```python
from build123d import *

# Parameters (mm, degrees)
SKETCH1_R            = 75
BOSS_EXTRUDE1_DEPTH  = 8
M5_CLEARANCE_HOLE1_D = 5.5
CUT_EXTRUDE2_DEPTH   = 4.2
SKETCH11_R           = 45.85
CUT_EXTRUDE3_DEPTH   = 6
SKETCH12_R           = 60.7695
SKETCH12_R_2         = 53.6575
CUT_EXTRUDE4_DEPTH   = 4.1656
SKETCH14_R           = 0.5
CENTER_HOLE_DEPTH    = 1


with BuildPart() as part:
    # Sketch1 → Boss-Extrude1 (new body)
    with BuildSketch(Plane.XY):
        Circle(SKETCH1_R)
    extrude(amount=BOSS_EXTRUDE1_DEPTH)

    # M5 Clearance Hole1 (through all)
    with Locations(Plane(origin=(0, 0, 0), x_dir=(-1, 0, 0), z_dir=(0, 0, -1))):
        with Locations((-17.470285544, -65.199993275), (-47.72970773, 47.72970773), (65.199993275, -17.470285544), (47.72970773, -47.72970773), (-65.199993275, 17.470285544), (-17.470285544, 65.199993275), (-65.199993275, -17.470285544), (-47.72970773, -47.72970773), (17.470285544, -65.199993275), (65.199993275, 17.470285544), (47.72970773, 47.72970773), (17.470285544, 65.199993275)):
            Hole(M5_CLEARANCE_HOLE1_D / 2)

    # Sketch6 → Cut-Extrude2 (cut)
    with BuildSketch(Plane(origin=(0, 0, 8), x_dir=(-1, 0, 0), z_dir=(0, 0, -1))):
        Polygon((-43.268287443, 46.534273767), (-44.463721406, 50.995694054), (-48.925141693, 52.191128017), (-52.191128017, 48.925141693), (-50.995694054, 44.463721406), (-46.534273767, 43.268287443), align=None)
        Polygon((-13.008865258, 66.395427237), (-16.274851582, 69.661413561), (-20.736271868, 68.465979598), (-21.931705831, 64.004559312), (-18.665719507, 60.738572988), (-14.204299221, 61.934006951), align=None)
        Polygon((21.931705831, 64.004559312), (20.736271868, 68.465979598), (16.274851582, 69.661413561), (13.008865258, 66.395427237), (14.204299221, 61.934006951), (18.665719507, 60.738572988), align=None)
        Polygon((50.995694054, 44.463721406), (52.191128017, 48.925141693), (48.925141693, 52.191128017), (44.463721406, 50.995694054), (43.268287443, 46.534273767), (46.534273767, 43.268287444), align=None)
        Polygon((66.395427237, 13.008865258), (69.661413561, 16.274851582), (68.465979598, 20.736271868), (64.004559312, 21.931705831), (60.738572988, 18.665719507), (61.934006951, 14.204299221), align=None)
        Polygon((64.004559312, -21.931705831), (68.465979598, -20.736271868), (69.661413561, -16.274851582), (66.395427237, -13.008865258), (61.934006951, -14.204299221), (60.738572988, -18.665719507), align=None)
        Polygon((44.463721406, -50.995694054), (48.925141693, -52.191128017), (52.191128017, -48.925141693), (50.995694054, -44.463721406), (46.534273767, -43.268287443), (43.268287444, -46.534273767), align=None)
        Polygon((13.008865258, -66.395427237), (16.274851582, -69.661413561), (20.736271868, -68.465979598), (21.931705831, -64.004559312), (18.665719507, -60.738572988), (14.204299221, -61.934006951), align=None)
        Polygon((-21.931705831, -64.004559312), (-20.736271868, -68.465979598), (-16.274851582, -69.661413561), (-13.008865258, -66.395427237), (-14.204299221, -61.934006951), (-18.665719507, -60.738572988), align=None)
        Polygon((-50.995694054, -44.463721406), (-52.191128017, -48.925141693), (-48.925141693, -52.191128017), (-44.463721406, -50.995694054), (-43.268287443, -46.534273767), (-46.534273767, -43.268287443), align=None)
        Polygon((-66.395427237, -13.008865258), (-69.661413561, -16.274851582), (-68.465979598, -20.736271868), (-64.004559312, -21.931705831), (-60.738572988, -18.665719507), (-61.934006951, -14.204299221), align=None)
        Polygon((-64.004559312, 21.931705831), (-68.465979598, 20.736271868), (-69.661413561, 16.274851582), (-66.395427237, 13.008865258), (-61.934006951, 14.204299221), (-60.738572988, 18.665719507), align=None)
    extrude(amount=CUT_EXTRUDE2_DEPTH, mode=Mode.SUBTRACT)

    # Sketch11 → Cut-Extrude3 (cut)
    with BuildSketch(Plane(origin=(0, 0, 0), x_dir=(-1, 0, 0), z_dir=(0, 0, -1))):
        Circle(SKETCH11_R)
    extrude(amount=-CUT_EXTRUDE3_DEPTH, mode=Mode.SUBTRACT)

    # Sketch12 → Cut-Extrude4 (cut)
    with BuildSketch(Plane(origin=(0, 0, 0), x_dir=(-1, 0, 0), z_dir=(0, 0, -1))):
        Circle(SKETCH12_R)
        Circle(SKETCH12_R_2, mode=Mode.SUBTRACT)
    extrude(amount=-CUT_EXTRUDE4_DEPTH, mode=Mode.SUBTRACT)

    # Sketch14 → center hole (cut)
    with BuildSketch(Plane.XY.offset(8)):
        Circle(SKETCH14_R)
    extrude(amount=-CENTER_HOLE_DEPTH, mode=Mode.SUBTRACT)


solid = part.part
```
For this review, take the finished solid that the model builds, in its own axes (mm). A direction names the side the tool comes from. Round coordinates to 2 decimals unless told otherwise and drop trailing zeros. Write each loop counter-clockwise with the first axis right and the second up, starting at its lowest first coordinate (ties: lowest second). Pieces come first, ordered by that corner, then holes. Notation, with made-up numbers: (-34, 87) - (2, 87) arc R7 ccw to (2, 91) - close; hole circle Ø5 at (-32, -4). An arc over 180 degrees is marked (long way). Use CSV: the item, a comma, the result in double quotes.
1) Add section A-A on z = 1.25. Count the separate pieces of the cut face and the enclosed holes in it, and give its area (3 significant figures).
Conclusion:
separate pieces,"2"
enclosed holes,"14"
area,"8,230 mm^2"
2) Clearance check with flat-ended pins moving along their axes: pin 1 Ø1.5 at (y, z) = (2, 1.5) entering from -X; pin 2 Ø2.5 at (x, y) = (-47, -48.5) entering from +Z; pin 3 Ø3 at (y, z) = (-24, 1) entering from -X; pin 4 Ø2 at (x, z) = (1, 4) entering from -Y. State where each tip first meets the part, or that it passes through.
Conclusion:
pin 1,"stops at x = -74.99"
pin 2,"passes through"
pin 3,"stops at x = -71.55"
pin 4,"stops at y = -75"
3) Add section C-C on x = 57.5. Write out the cut boundary in (y, z).
Conclusion:
outline,"(-48.15, 0) - (-19.66, 0) - (-19.66, 4.17) - (19.66, 4.17) - (19.66, 0) - (48.15, 0) - (48.15, 8) - (-48.15, 8) - close"
4) The part is to be moulded in two halves that separate along X. For faces 3 (the flat face through (-61.345, -16.404, 5.929)), 4 (the flat face through (-1, 1, 8)), say which applies: pulls with the +X half, pulls with the -X half, needs draft (parallel to the pull), parting line crosses it, or undercut.
Conclusion:
face 3,"undercut"
face 4,"needs draft"
5) Add section D-D on x = -24.5. Write out the cut boundary in (y, z), and give its area (4 significant figures).
Conclusion:
outline,"(-70.89, 0) - (-55.61, 0) - (-55.61, 4.17) - (-47.74, 4.17) - (-47.74, 0) - (-38.76, 0) - (-38.76, 6) - (38.76, 6) - (38.76, 0) - (47.74, 0) - (47.74, 4.17) - (55.61, 4.17) - (55.61, 0) - (70.89, 0) - (70.89, 8) - (-70.89, 8) - close"
area,"603.5 mm^2"
6) Wall thickness on line 1 along X through (y, z) = (-49, 4.5); line 2 along Y through (x, z) = (46.5, 5.5); line 3 along X through (y, z) = (27, 1.25): over which ranges is each line inside the solid? List them lowest first. Write a range as from..to.
Conclusion:
line 1,"x = -56.78..-52.12, -43.93..43.93, 52.12..56.78"
line 2,"y = -58.85..-51.54, -43.3..43.3, 51.54..58.85"
line 3,"x = -69.97..-54.44, -46.37..-37.06, 37.06..46.37, 54.44..69.97"
7) For faces 1 (the cylindrical face through (-50.477, -47.609, 1.927)), 2 (the flat face through (50.581, -50.535, 5.929)), list the 3-axis set-ups (+Z, -Z, +X, -X, +Y, -Y) from which the entire face can be reached by the end or side of a thin tool; tool diameter is ignored.
Conclusion:
face 1,"+Z, -Z"
face 2,"+Z"
8) Add section B-B on y = 24. Write out the cut boundary in (x, z).
Conclusion:
outline,"(-71.06, 0) - (-55.83, 0) - (-55.83, 4.17) - (-47.99, 4.17) - (-47.99, 0) - (-39.07, 0) - (-39.07, 6) - (39.07, 6) - (39.07, 0) - (47.99, 0) - (47.99, 4.17) - (55.83, 4.17) - (55.83, 0) - (71.06, 0) - (71.06, 8) - (-71.06, 8) - close"
